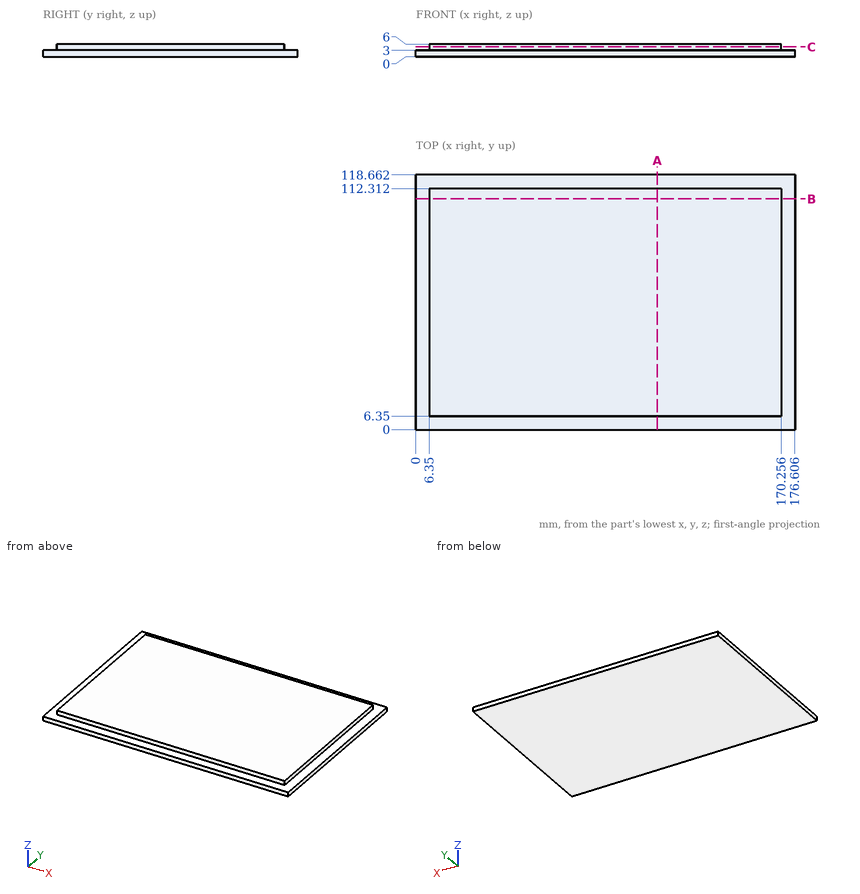
Study the drawing (mm; zero at the part's minimum x, y, z) and answer. Coordinates: 2 decimals unless noted, no trailing zeros. Write each loop counter-clockwise with the first axis right and the second up, starting at its lowest first coordinate (ties: lowest second). Pieces come first, ordered by that corner, then holes. Notation, with made-up numbers: M 88.5,36 L 133.5,36 A20 cw 133.5,72 Z; hole C -20.75,81.25 d8. An arc over 180 degrees is marked long. Use a Markdown table: item, result. Add a question column.
1. Section A-A (x = 112.5) is taken. Give the vertices of the cut face in (y, z), plus the area to 3 significant figures.
2. Given P1, Ø0.9, axis at y = 65.5, z = 4.5, coming from the -X side; P2, Ø1.5, axis at y = 64.5, z = 4, coming from the +X side; P3, Ø2.5, axis at x = 108.5, z = 5, coming from the -Y side, each flat-ended and moving along its own axis, determine where each tip first touches the part or whether it passes through.
3. Section B-B (y = 107.5) is taken. Give the vertices of the cut face in (x, z), plus the area to 3 significant figures.
4. Straight lines are drawn through the part: line 1 along X through (y, z) = (97, 5.65); line 2 along Y through (x, z) = (139, 5.35). For each, find the intervals that lie inside material, in ascending order. Write a range as [from, to].
5. Section C-C (z = 4.7) is taken. Give the vertices of the cut face in (x, y).
Data:
| question | item | result |
|---|---|---|
| 1 | outline | M 0,0 L 118.66,0 L 118.66,3 L 112.31,3 L 112.31,6 L 6.35,6 L 6.35,3 L 0,3 Z |
| 1 | area | 674 mm2 |
| 2 | P1 | stops at x = 6.35 |
| 2 | P2 | stops at x = 170.26 |
| 2 | P3 | stops at y = 6.35 |
| 3 | outline | M 0,0 L 176.61,0 L 176.61,3 L 170.26,3 L 170.26,6 L 6.35,6 L 6.35,3 L 0,3 Z |
| 3 | area | 1,020 mm2 |
| 4 | line 1 | x = [6.35, 170.26] |
| 4 | line 2 | y = [6.35, 112.31] |
| 5 | outline | M 6.35,6.35 L 170.26,6.35 L 170.26,112.31 L 6.35,112.31 Z |
